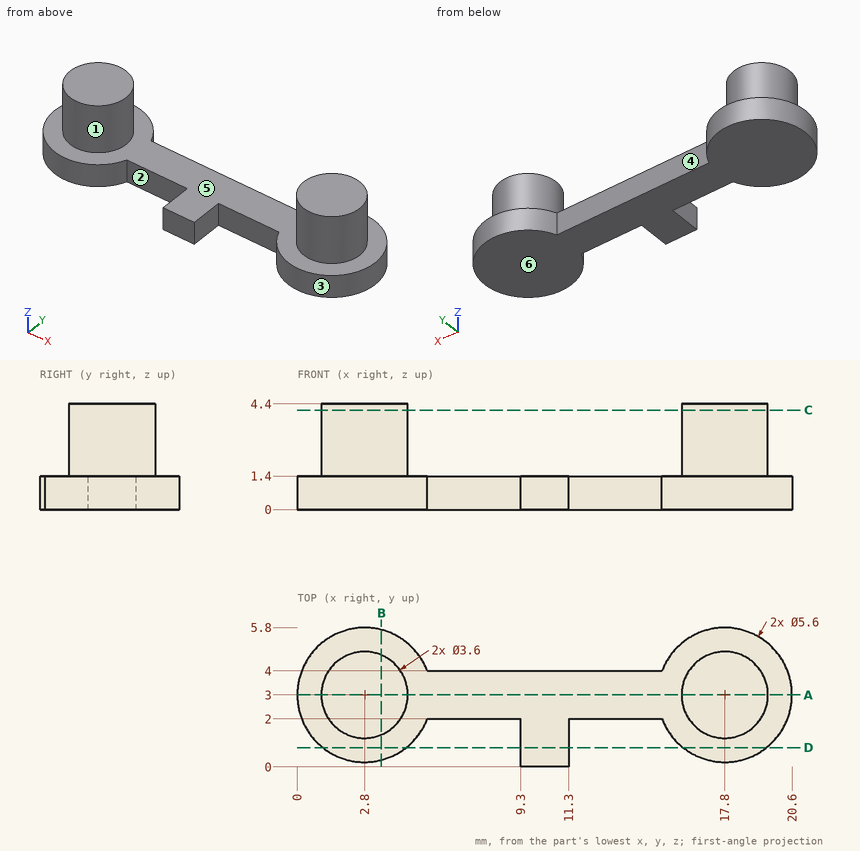
The figure shows three views and two pictorial views of one solid part (mm, origin at its lowest corner). Answer the questions. A direction names the side the tool comes from. Round coordinates to 2 decimals unless told otherwise and drop trailing zeros. Write each loop counter-clockwise with the first axis right and the second up, starting at its lowest first coordinate (ties: lowest second). Pieces come first, ordered by that corner, then holes. Notation, with made-up numbers: (-35.75, 33.25) - (0.25, 33.25) arc R13 cw to (0.25, 46.25) - close; hole circle Ø11 at (-21.5, 84). An arc over 180 degrees is marked (long way). Answer in a Markdown table with one row per item. Add a question column.
1. A cutting plane is placed at D-D, the plane y = 0.8. Determine the outline of the cut face in (x, z), and give its area (3 significant figures).
2. For the marked faces 1, 2, 3 and 4, determine the directions among +Z, -Z, +X, -X, +Y, -Y from which every point of the face is accessible in a straight line to the end or side of a thin tool.
3. Find the intervals of material crossed by line 1 along X through (y, z) = (1.35, 1.1); line 2 along X through (y, z) = (1, 1.2); line 3 along Y through (x, z) = (10.75, 0.65), in increasing order. Write a range as from..to.
4. A cutting plane is placed at C-C, the plane z = 4.15. Determine the outline of the cut face in (x, y).
5. A cutting plane is placed at B-B, the plane x = 3.5. Determine the outline of the cut face in (y, z), and give its area (3 significant figures).
6. Given pin 1 (2 mm diameter, centred on x = 10.5, z = 0.5, fed in from +Y); pin 2 (1.7 mm diameter, centred on x = 6, y = 1.5, fed in from +Z); pin 3 (1.5 mm diameter, centred on y = 1, z = 1, fed in from +X), each flat-ended and moving along its own axis, determine where each tip first touches the part or whether it passes through.
7. The mould has two halves that part along X. Classify the marked faces 5 and 6: +X half, -X half, draft (parallel to the pull), parting line (faces both ways), or undercut.
8. A cutting plane is placed at A-A, the plane y = 3. Determine the outline of the cut face in (x, z), and give its area (3 significant figures).
Worked out:
| question | item | result |
|---|---|---|
| 1 | outline | (1.07, 0) - (4.53, 0) - (4.53, 1.4) - (1.07, 1.4) - close; (9.3, 0) - (11.3, 0) - (11.3, 1.4) - (9.3, 1.4) - close; (16.07, 0) - (19.53, 0) - (19.53, 1.4) - (16.07, 1.4) - close |
| 1 | area | 12.5 mm^2 |
| 2 | face 1 | +Z |
| 2 | face 2 | +Z, -Z, -Y |
| 2 | face 3 | +Z, -Z |
| 2 | face 4 | +Z, -Z, +Y |
| 3 | line 1 | 0.54..5.06, 9.3..11.3, 15.54..20.06 |
| 3 | line 2 | 0.84..4.76, 9.3..11.3, 15.84..19.76 |
| 3 | line 3 | 0..4 |
| 4 | outline | circle Ø3.6 at (2.8, 3); circle Ø3.6 at (17.8, 3) |
| 5 | outline | (0.29, 0) - (5.71, 0) - (5.71, 1.4) - (4.66, 1.4) - (4.66, 4.4) - (1.34, 4.4) - (1.34, 1.4) - (0.29, 1.4) - close |
| 5 | area | 17.5 mm^2 |
| 6 | pin 1 | y = 4 |
| 6 | pin 2 | z = 1.4 |
| 6 | pin 3 | x = 20.31 |
| 7 | face 5 | undercut |
| 7 | face 6 | draft |
| 8 | outline | (0, 0) - (20.6, 0) - (20.6, 1.4) - (19.6, 1.4) - (19.6, 4.4) - (16, 4.4) - (16, 1.4) - (4.6, 1.4) - (4.6, 4.4) - (1, 4.4) - (1, 1.4) - (0, 1.4) - close |
| 8 | area | 50.4 mm^2 |
